Part model, mm, in its own coordinate system. A direction names the side the tool comes from. Round coordinates to 2 decimals unless told otherwise and drop trailing zeros. Write each loop counter-clockwise with the first axis right and the second up, starting at its lowest first coordinate (ties: lowest second). Pieces come first, ordered by that corner, then holes. Notation, with made-up numbers: M 66,60.25 L 118,60.25 A27 ccw 118,81.25 Z; hole C -30.5,19 d6. An arc over 180 degrees is marked long. Use one line per item in the form item = value. Start each with the question number.
Item 1: Cut at A-A, the plane x = 0. Give the cut face in (y, z).
Item 2: Cut at C-C, the plane z = 17.25. Give the cut face in (x, y).
Item 3: Cut at B-B, the plane y = 0. Give the cut face in (x, z), then the cut area to 3 significant figures.
Item 4: Probe L1, parallel to Y at x = 0, z = 6.75; L2, parallel to Y at x = 2, z = 26.5; L3, parallel to Y at x = -6, z = 10. List the from-to ranges inside material, lowest first.
Item 5: Mould opens along Y. For faces 3 (the face through (-2.44, -18.59, 14.8)), 4 (the face through (0, 6, 15)), 5 (the face through (4, -4, 30)) say: +Y half, -Y half, draft (parallel to the pull), parting line (faces both ways), or undercut.
Item 6: Flat gauge pins, fed straight in: pin 1 Ø1 at (y, z) = (5.5, 10) entering from +X; pin 2 Ø3.5 at (x, z) = (-0.5, 10.5) entering from -Y; pin 3 Ø10 at (y, z) = (-0.5, 15.5) entering from -X; pin 4 Ø6 at (x, y) = (0, 0) entering from +Z. Where does each tip first touch, or does it go through?
Item 7: Which spindle directions (+Z, -Z, +X, -X, +Y, -Y) get a long thin tool onto all of the face, cutting with end or side? Do faces 1 (the face through (1.5, 5, 15)), 2 (the face through (4, -4, 0)). Say none if no direction does.
Solid Edge part; units mm, degrees
sketch "Sketch1" plane through (0, 0, 0) normal (0, 0, 1) x (1, 0, 0)
  circle A0 centre (0, 0) radius 18.75
extrude "Protrusion1" add sketch "Sketch1" along normal blind 30
sketch "Sketch2" plane through (0, 0, 30) normal (0, 0, 1) x (1, 0, 0)
  circle A0 centre (0, 0) radius 5
  line L0 (-1.5, 4) -> (1.5, 4)
  line L1 (1.5, 4) -> (1.5, 6)
  line L2 (1.5, 6) -> (-1.5, 6)
  line L3 (-1.5, 6) -> (-1.5, 4)
extrude "Cutout1" cut sketch "Sketch2" against normal through all
fillet "Round_1" radius 1 2 edges at (-18.75, 0, 30) (-18.75, 0, 0)
properties material "Stainless steel"
Model answer:
q1.outline = M -18.75,1 A1 ccw -17.75,0 L -5,0 L -5,30 L -17.75,30 A1 ccw -18.75,29 Z; M 6,0 L 17.75,0 A1 ccw 18.75,1 L 18.75,29 A1 ccw 17.75,30 L 6,30 Z
q2.outline = C 0,0 d37.5; hole M -1.5,4.77 A5 ccw long 1.5,4.77 L 1.5,6 L -1.5,6 Z
q3.outline = M -18.75,1 A1 ccw -17.75,0 L -5,0 L -5,30 L -17.75,30 A1 ccw -18.75,29 Z; M 5,0 L 17.75,0 A1 ccw 18.75,1 L 18.75,29 A1 ccw 17.75,30 L 5,30 Z
q3.area = 824 mm²
q4.L1 = -18.75 to -5, 6 to 18.75
q4.L2 = -18.64 to -4.58, 4.58 to 18.64
q4.L3 = -17.76 to 17.76
q5.face_3 = parting line
q5.face_4 = undercut
q5.face_5 = draft
q6.pin_1 = 18.07
q6.pin_2 = -18.75
q6.pin_3 = -18.75
q6.pin_4 = through
q7.face_1 = +Z, -Z
q7.face_2 = -Z, +X, -X, +Y, -Y
